```python
from build123d import *

# Parameters (mm, degrees)
F1_R     = 3
F2_DEPTH = 8
F3_SIZE2 = 0.2679491924
F3_SIZE  = 1
F4_W     = 6
F4_H     = 6
F5_DEPTH = 8


with BuildPart() as f2:
    # F1 (on Front) → F2 (new body, symmetric)
    with BuildSketch(Plane.XZ):
        Circle(F1_R)
    extrude(amount=F2_DEPTH, both=True)

    # F3
    f3_edges = [f2.edges().sort_by_distance(p)[0] for p in [
        (-3, -8, 0),
        (-3, 8, 0),
    ]]
    f3_side = f2.faces().sort_by_distance((-3, 0, 0))[0]
    chamfer(f3_edges, length=F3_SIZE, length2=F3_SIZE2, reference=f3_side)

    # F4 (on Front) → F5 (cut, symmetric)
    with BuildSketch(Plane.XZ):
        with Locations((0, 5.55)):
            Rectangle(F4_W, F4_H)
    extrude(amount=F5_DEPTH, both=True, mode=Mode.SUBTRACT)


solid = f2.part
```
Source: CAD feature listing. Evaluate the final solid. Frame: model axes, mm. Round coordinates to 2 decimals unless told otherwise and drop trailing zeros. Loops run counter-clockwise (first coordinate to the right, second up) from the corner with the lowest first, then second, coordinate; pieces in that order, holes last. Notation, with made-up numbers: M 58,-34.5 L 103,-34.5 A32 ccw 103,-1.5 Z; hole C -38,72 d2. An arc over 180 degrees is marked long. Use a Markdown table: item, result. Add a question column.
1. Section query A-A on y = 3.25. Return the cut outline in (x, z).
2. Line query: line 1 (X direction, y = 1.75, z = -0.15); line 2 (Z direction, x = 1.25, y = 2); line 3 (X direction, y = 5.75, z = 0.95). Output: solid intervals per line, ascending.
3. Contact query for flat-ended pins moving along their axis: P1, Ø3, axis at y = -1, z = -0.5, coming from the +X side; P2, Ø2, axis at x = -2, y = -0.5, coming from the -Z side. Output: stop coordinate, or through.
Reported:
| question | item | result |
|---|---|---|
| 1 | outline | M -1.58,2.55 A3 ccw long 1.58,2.55 Z |
| 2 | line 1 | x = -3 to 3 |
| 2 | line 2 | z = -2.73 to 2.55 |
| 2 | line 3 | x = -2.85 to 2.85 |
| 3 | P1 | stops at x = 3 |
| 3 | P2 | stops at z = -2.83 |
